```python
from build123d import *

# Parameters (mm, degrees)
SKETCH1_W           = 26
SKETCH1_H           = 12
SKETCH1_R           = 1.25
BOSS_EXTRUDE1_DEPTH = 1.5
SKETCH2_W           = 17
SKETCH2_H           = 5
BOSS_EXTRUDE2_DEPTH = 2.2
SKETCH2_3_W         = 7.5
SKETCH2_3_H         = 4.5
BOSS_EXTRUDE3_DEPTH = 3
SKETCH3_W           = 7.1
SKETCH3_H           = 2.6
CUT_EXTRUDE1_DEPTH  = 4.3
SKETCH4_W           = 16.6
SKETCH4_H           = 1.8
CUT_EXTRUDE2_DEPTH  = 4.8
SKETCH5_W           = 6.5
SKETCH5_H           = 4
BOSS_EXTRUDE4_DEPTH = 0.8


with BuildPart() as part:
    # Sketch1 → Boss-Extrude1 (new body)
    with BuildSketch(Plane(origin=(0, 0, 0), x_dir=(1, 0, 0), z_dir=(0, 1, 0))):
        with Locations((13, 6)):
            Rectangle(SKETCH1_W, SKETCH1_H)
        with Locations(Location((1.55, 10.45, 0), (0, 0, 270))):
            Circle(SKETCH1_R, mode=Mode.SUBTRACT)
        with Locations(Location((24.45, 1.55, 0), (0, 0, 270))):
            Circle(SKETCH1_R, mode=Mode.SUBTRACT)
    extrude(amount=BOSS_EXTRUDE1_DEPTH)

    # Sketch2 → Boss-Extrude2 (add)
    with BuildSketch(Plane(origin=(0, 1.5, 0), x_dir=(1, 0, 0), z_dir=(0, 1, 0))):
        with Locations((9.5, 2.7)):
            Rectangle(SKETCH2_W, SKETCH2_H)
    extrude(amount=BOSS_EXTRUDE2_DEPTH)

    # Sketch2<3> → Boss-Extrude3 (add)
    with BuildSketch(Plane(origin=(0, 1.5, 0), x_dir=(1, 0, 0), z_dir=(0, 1, 0))):
        with Locations((19.25, 9.55)):
            Rectangle(SKETCH2_3_W, SKETCH2_3_H)
    extrude(amount=BOSS_EXTRUDE3_DEPTH)

    # Sketch3 → Cut-Extrude1 (cut)
    with BuildSketch(Plane(origin=(0, 0, -11.8), x_dir=(-1, 0, 0), z_dir=(0, 0, -1))):
        with Locations((-19.25, 3)):
            Rectangle(SKETCH3_W, SKETCH3_H)
    extrude(amount=-CUT_EXTRUDE1_DEPTH, mode=Mode.SUBTRACT)

    # Sketch4 → Cut-Extrude2 (cut)
    with BuildSketch(Plane.XY.offset(-0.2)):
        with Locations((9.5, 2.6)):
            Rectangle(SKETCH4_W, SKETCH4_H)
    extrude(amount=-CUT_EXTRUDE2_DEPTH, mode=Mode.SUBTRACT)

    # Sketch5 → Boss-Extrude4 (add)
    with BuildSketch(Plane.XZ):
        with Locations((9.25, -8.6)):
            Rectangle(SKETCH5_W, SKETCH5_H)
    extrude(amount=BOSS_EXTRUDE4_DEPTH)


solid = part.part
```
Verification items for the finished model (mm, model axes). A direction names the side the tool comes from. Round coordinates to 2 decimals unless told otherwise and drop trailing zeros. Write each loop counter-clockwise with the first axis right and the second up, starting at its lowest first coordinate (ties: lowest second). Pieces come first, ordered by that corner, then holes. Notation, with made-up numbers: (18, -3.75) -> (52, -3.75) arc R28 cw to (52, 29.25) -> close; hole circle Ø9 at (72.25, -3.75). An arc over 180 degrees is marked (long way). Write each question's results on one line, items separated by ' | '.
Q1. Access from +Z, -Z, +X, -X, +Y, -Y to the whole of each face (thin tool, end or side, straight path). Record for faces 1 (the face through (18, 3, -3)), 2 (the face through (19, 4.3, -10)), 3 (the face through (19, 3, -7.3)), 4 (the face through (1.2, 3, -3)).
Derived:
face 1: +Z, +X, +Y | face 2: -Z | face 3: +X, -X, +Y | face 4: +Z
Q2. Thickness scan on probe 1 along Y at (x, z) = (16, -4.5); probe 2 along X at (y, z) = (1.9, -8.75); probe 3 along Z at (x, y) = (1.5, 0.5). Record the ranges inside material, lowest first.
Derived:
probe 1: y = 0 to 1.7, 3.5 to 3.7 | probe 2: x = 15.5 to 15.7, 22.8 to 23 | probe 3: z = -12 to -11.7, -9.2 to 0
Q3. Sectioned sample at D-D, the plane z = -4. Record the boundary of the cut face in (x, y).
Derived:
outline: (0, 0) -> (26, 0) -> (26, 1.5) -> (18, 1.5) -> (18, 3.7) -> (1, 3.7) -> (1, 1.5) -> (0, 1.5) -> close; hole (1.2, 1.7) -> (17.8, 1.7) -> (17.8, 3.5) -> (1.2, 3.5) -> close
Q4. Go/stop test with flat-tipped pins: pin 1 Ø1.1 at (x, y) = (6.5, 2.5) entering from -Z; pin 2 Ø0.9 at (y, z) = (-0.5, -7.5) entering from -X; pin 3 Ø0.9 at (y, z) = (-0.5, -7.5) entering from +X. Record where each tip stops, or that it passes through.
Derived:
pin 1: stops at z = -5.2 | pin 2: stops at x = 6 | pin 3: stops at x = 12.5
Q5. Sectioned sample at B-B, the plane x = 24.45. Record the boundary of the cut face in (y, z).
Derived:
outline: (0, -12) -> (1.5, -12) -> (1.5, -2.8) -> (0, -2.8) -> close; (0, -0.3) -> (1.5, -0.3) -> (1.5, 0) -> (0, 0) -> close
Q6. Draft check along X on faces 5 (the face through (17.8, 3, -3)), 6 (the face through (9, -0.8, -9)), 7 (the face through (15.5, 3, -10)). Enter one of: released by +X, released by -X, zero draft, split by the parting line, or undercut.
Derived:
face 5: undercut | face 6: zero draft | face 7: released by -X
Q7. Sectioned sample at A-A, the plane z = -1.55. Record the boundary of the cut face in (x, y), and give its area (3 significant figures).
Derived:
outline: (0, 0) -> (23.2, 0) -> (23.2, 1.5) -> (18, 1.5) -> (18, 3.7) -> (1, 3.7) -> (1, 1.5) -> (0, 1.5) -> close; (25.7, 0) -> (26, 0) -> (26, 1.5) -> (25.7, 1.5) -> close; hole (1.2, 1.7) -> (17.8, 1.7) -> (17.8, 3.5) -> (1.2, 3.5) -> close | area: 42.8 mm²
Q8. Sectioned sample at C-C, the plane y = 2.15. Record the boundary of the cut face in (x, z).
Derived:
outline: (1, -5.2) -> (18, -5.2) -> (18, -0.2) -> (17.8, -0.2) -> (17.8, -5) -> (1.2, -5) -> (1.2, -0.2) -> (1, -0.2) -> close; (15.5, -11.8) -> (15.7, -11.8) -> (15.7, -7.5) -> (22.8, -7.5) -> (22.8, -11.8) -> (23, -11.8) -> (23, -7.3) -> (15.5, -7.3) -> close
